Design review of the part built by this model. Coordinates are the model's own, in mm. A direction names the side the tool comes from. Coordinates: 2 decimals unless noted, no trailing zeros. Order: outer loops, then holes, each group sorted by start corner. A loop starts at its lowest first (then second) coordinate and runs counter-clockwise, first axis right, second up. Notation, with made-up numbers: (9, 63.25) - (18, 63.25) arc R26 cw to (18, 86.25) - close; hole circle Ø9 at (44, 10.25). An arc over 180 degrees is marked (long way). Write each question's results on one line, items separated by ' | '. Start each with the question number.
Autodesk Inventor part; units mm, degrees
ref_plane "Work Plane1" through (23.5, 0, 0) normal (1, 0, 0) x (0, 1, 0)
ref_plane "XZ Plane" through (0, 0, 0) normal (0, 1, 0) x (-1, 0, 0)
ref_plane "XY Plane" through (0, 0, 0) normal (0, 0, 1) x (1, 0, 0)
sketch "Sketch1" plane through (0, 0, 0) normal (0, 0, 1) x (1, 0, 0)
  line L0 (-23.5, -52.5) -> (23.5, -52.5)
  line L1 (23.5, -52.5) -> (23.5, 52.5)
  line L2 (23.5, 52.5) -> (-23.5, 52.5)
  line L3 (-23.5, 52.5) -> (-23.5, -52.5)
  line L4 (-23.5, -52.5) -> (23.5, 52.5) construction
  line L5 (23.5, -52.5) -> (-23.5, 52.5) construction
  line L6 (-23.5, 12) -> (17, 52.5)
  line L7 (-20, -52.5) -> (23.5, -9)
  line L8 (21.5, 52.5) -> (21.5, -52.5)
  line L9 (-21.5, 52.5) -> (-21.5, -52.5)
  line L10 (0, 52.5) -> (0, 7) construction
  line L11 (-7, 52.5) -> (-7, 7)
  line L12 (7, 7) -> (7, 52.5)
  arc A0 (7, 52.5) -> (-7, 52.5) centre (0, 52.5) ccw
  arc A1 (-7, 7) -> (7, 7) centre (0, 7) ccw
  line L13 (0, 52.5) -> (0, -52.5)
  line L14 (0, -74.9) -> (0, 81.9)
  point P0 (0, 0)
  point P1 (0, 29.75)
  point P2 (7, 52.5)
  point P3 (-7, 52.5)
  point P4 (-7, 28.5)
  point P5 (7, 42.5)
  dimension "d0" = 2
  dimension "d1" = 2
  dimension "d2" = 47
  dimension "d3" = 14
  dimension "d4" = 105
  dimension "d5" = 52.5
  dimension "d6" = 20
  dimension "d7" = 45
  dimension "d9" = 17
revolve "Revolution1" add sketch "Sketch1" angle 360 about axis through (0, -10, 0) along (0, 1, 0) contours L8 L7 L1 L0 | L8 L2 L1 L7
extrude "Extrusion1" cut sketch "Sketch1" along normal through all both and the other way through all contours L3 L2 L9 L6 | L7 L13 L0 | L9 L2 L11 L6 | L13 L7 L8 L0 | L11 L2 L13 L6 | L6 L13 A1 L11 | L8 L7 L1 L0 | L13 L6 L12 A1 | L13 L2 L12 L6 | A0 L14 L2 | L12 L2 L6 | L14 A0 L2
ref_plane "Work Plane1" through (23.5, 0, 0) normal (1, 0, 0) x (0, 1, 0)
sketch "Sketch2" plane through (23.5, 0, 0) normal (1, 0, 0) x (0, 1, 0)
  arc A0 (52.5, -16.225) -> (42.5, 22.4332) centre (35.5, 0) ccw
  line L0 (42.5, 22.4332) -> (7, 22.4332)
  line L1 (7, 22.4332) -> (28.5, 22.4332)
  arc A1 (28.5, 22.4332) -> (28.5, -22.4332) centre (35.5, 0) ccw
  line L2 (28.5, -22.4332) -> (7, -22.4332)
  line L3 (7, -22.4332) -> (42.5, -22.4332)
  arc A2 (42.5, -22.4332) -> (52.5, 16.225) centre (35.5, 0) ccw
  line L4 (52.5, 16.225) -> (52.5, -16.225)
  arc A3 (-52.5, -12.339) -> (-52.5, 12.339) centre (-32.5, 0) ccw
  line L5 (-52.5, 12.339) -> (-52.5, -12.339)
  line L6 (52.5, -16.225) -> (52.5, 16.225)
  line L7 (52.5, 0) -> (-9, 0)
  arc A4 (-52.5, -12.339) -> (-52.5, 12.339) centre (-32.5, 0) ccw
  point P0 (0, 0)
  point P1 (12, 0)
  point P2 (7, 0)
  dimension "d20" = 5
hole "Hole1" at (23.5, 7, 0) direction (-1, 0, 0) diameter 2.9 depth 5 counterbore diameter 5.5 counterbore depth 0.5
equation "\"d1\" = d0"
properties part number "Test_Blade_Guard"
(1) Mouldability with a two-part tool opening along Y and no side actions: class faces 4 (the face through (-22, -52.5, 0)), 5 (the face through (23, 8.2, -1.2)), 6 (the face through (-23.477, 0.735, -1.033)) as +Y half, -Y half, draft (parallel to the pull), parting line (faces both ways), or undercut.
(2) Take a section at A-A (z = 0). State the section outline as (x, y) points.
(3) Take a section at D-D (z = -9.5). State the section outline as (x, y) points.
(4) Clearance check with flat-ended pins moving along their axes: pin 1 (1.1 mm diameter, centred on y = 14, z = 21, fed in from +X); pin 2 (2 mm diameter, centred on x = -14.5, y = -7, fed in from +Z); pin 3 (1.1 mm diameter, centred on y = 32.5, z = 21, fed in from -X); pin 4 (6.5 mm diameter, centred on y = 7, z = 0, fed in from +X). State where each tip first meets the part, or that it passes through.
(5) Take a section at B-B (x = 0). State the section outline as (y, z) points.
(6) Tool access review of faces 1 (the face through (22.215, 8.286, -0.669)), 2 (the face through (-7, 18, -21)), 3 (the face through (12.3, 47.8, 18.5)): name each direction out of +Z, -Z, +X, -X, +Y, -Y from which nothing blocks a thin tool from reaching the whole face with its end or side.
(7) To check wall thickness, follow line 1 along Z through (x, y) = (0, -29.5); line 2 along X through (y, z) = (-14.5, -0.5). State the ranges of each line that lie inside material, in increasing order. Write a range as [from, to].
(8) Take a section at C-C (y = 13). State the section outline as (x, z) points, plus the area to 3 significant figures.
Worked out:
1) face 4: -Y half | face 5: undercut | face 6: draft
2) outline: (-23.5, -52.5) - (-21.5, -52.5) - (-21.5, 14) - (-23.5, 12) - close; (21.5, -11) - (23.5, -9) - (23.5, 4.25) - (23, 4.25) - (23, 5.55) - (21.5, 5.55) - close; (21.5, 8.45) - (23, 8.45) - (23, 9.75) - (23.5, 9.75) - (23.5, 52.5) - (21.5, 52.5) - close
3) outline: (-21.49, -52.5) - (-20, -52.5) - (-19.29, -51.79) - (-19.29, 16.21) - (-21.49, 14.01) - close; (19.29, -13.21) - (21.49, -11.01) - (21.49, 52.5) - (19.29, 52.5) - close
4) pin 1: x = 11.58 | pin 2: z = 19.24 | pin 3: x = 7 | pin 4: x = 23.5
5) outline: (-32.5, -23.5) - (0, -23.5) - (0, -21.5) - (-32.5, -21.5) - close; (-32.5, 21.5) - (0, 21.5) - (0, 23.5) - (-32.5, 23.5) - close
6) face 1: +X | face 2: +Z, -Z, +Y | face 3: +Z, -Z, -X, +Y
7) line 1: [-23.5, -21.5], [21.5, 23.5] | line 2: [-23.49, -21.49]
8) outline: (-22.5, -6.78) arc R23.5 ccw to (-7, -22.43) - (-7, -20.33) arc R21.5 cw to (-7, 20.33) - (-7, 22.43) arc R23.5 ccw to (-22.5, 6.78) - close; (7, -22.43) arc R23.5 ccw to (7, 22.43) - (7, 20.33) arc R21.5 cw to (7, -20.33) - close | area: 217 mm^2
